Model file for the job. Use its own axes, mm. A direction names the side the tool comes from. Coordinates: 2 decimals unless noted, no trailing zeros. Loops run counter-clockwise (first coordinate to the right, second up) from the corner with the lowest first, then second, coordinate; pieces in that order, holes last. Notation, with made-up numbers: (79, 52) -> (131, 52) arc R18 cw to (131, 63) -> close; hole circle Ø5 at (33, 55). An arc over 180 degrees is marked (long way). Use one line per item in the form item = value.
```python
from build123d import *

# Parameters (mm, degrees)
EXTRUDE_1_DEPTH = 10
SHELL_2_T       = 3
FILLET_3_R      = 10
FILLET_4_R      = 3
SKETCH_2_R      = 2.675
EXTRUDE_2_DEPTH = 8
FILLET_7_R      = 5
CHAMFER_1_SIZE  = 0.2
CHAMFER_2_SIZE  = 0.2
FILLET_9_SIZE   = 5.5
FILLET_9_SIZE_2 = 5


# Some blends are built 0.0001 mm under size
with BuildPart() as part:
    # 草图1 → 凸台-拉伸1 (new body)
    with BuildSketch(Plane(origin=(0, 0, 0), x_dir=(1, 0, 0), z_dir=(0, 1, 0))):
        with BuildLine():
            Line((-37.5, 15), (37.5, 15))
            ThreePointArc((37.5, 15), (44.571067812, 12.071067812), (47.5, 5))
            Line((47.5, 5), (47.5, -5))
            ThreePointArc((47.5, -5), (44.571067812, -12.071067812), (37.5, -15))
            Line((37.5, -15), (-37.5, -15))
            ThreePointArc((-37.5, -15), (-44.571067812, -12.071067812), (-47.5, -5))
            Line((-47.5, -5), (-47.5, 5))
            ThreePointArc((-47.5, 5), (-44.571067812, 12.071067812), (-37.5, 15))
        make_face()
    extrude(amount=EXTRUDE_1_DEPTH)

    # 抽壳2
    shell_2_openings = [part.faces().sort_by_distance(p)[0] for p in [
        (0, 0, 0),
    ]]
    offset(amount=SHELL_2_T, openings=shell_2_openings, kind=Kind.INTERSECTION)

    # 圆角3
    # the kernel refuses this fillet: 10 mm, written as the material it takes off along each edge
    with BuildSketch(Plane(origin=(37.5, 13, 5), x_dir=(1, 0, 0), z_dir=(0, 0, -1))) as fillet_3_piece_1:
        with BuildLine():
            CenterArc((13 - FILLET_3_R, FILLET_3_R), FILLET_3_R, 270, 90)
            Line((13 - FILLET_3_R, 0), (13, 0))
            Line((13, 0), (13, FILLET_3_R))
        make_face()
    revolve(axis=Axis((37.5, 13, 5), (0, -1, 0)), revolution_arc=90, mode=Mode.SUBTRACT)
    with BuildSketch(Plane(origin=(50.5, 13, 5), x_dir=(0, -1, 0), z_dir=(0, 0, -1)), Plane(origin=(-50.5, 13, -5), x_dir=(0, -1, 0), z_dir=(0, 0, 1))) as fillet_3_piece_2:
        with BuildLine():
            CenterArc((FILLET_3_R, FILLET_3_R), FILLET_3_R, 180, 90)
            Line((0, FILLET_3_R), (0, 0))
            Line((0, 0), (FILLET_3_R, 0))
        make_face()
    extrude(amount=10, mode=Mode.SUBTRACT)
    with BuildSketch(Plane(origin=(37.5, 13, -5), x_dir=(0, 0, -1), z_dir=(-1, 0, 0))) as fillet_3_piece_3:
        with BuildLine():
            CenterArc((13 - FILLET_3_R, FILLET_3_R), FILLET_3_R, 270, 90)
            Line((13 - FILLET_3_R, 0), (13, 0))
            Line((13, 0), (13, FILLET_3_R))
        make_face()
    revolve(axis=Axis((37.5, 13, -5), (0, -1, 0)), revolution_arc=90, mode=Mode.SUBTRACT)
    with BuildSketch(Plane(origin=(37.5, 13, -18), x_dir=(0, -1, 0), z_dir=(-1, 0, 0)), Plane(origin=(-37.5, 13, 18), x_dir=(0, -1, 0), z_dir=(1, 0, 0))) as fillet_3_piece_4:
        with BuildLine():
            CenterArc((FILLET_3_R, FILLET_3_R), FILLET_3_R, 180, 90)
            Line((0, FILLET_3_R), (0, 0))
            Line((0, 0), (FILLET_3_R, 0))
        make_face()
    extrude(amount=75, mode=Mode.SUBTRACT)
    with BuildSketch(Plane(origin=(-37.5, 13, -5), x_dir=(-1, 0, 0), z_dir=(0, 0, 1))) as fillet_3_piece_5:
        with BuildLine():
            CenterArc((13 - FILLET_3_R, FILLET_3_R), FILLET_3_R, 270, 90)
            Line((13 - FILLET_3_R, 0), (13, 0))
            Line((13, 0), (13, FILLET_3_R))
        make_face()
    revolve(axis=Axis((-37.5, 13, -5), (0, -1, 0)), revolution_arc=90, mode=Mode.SUBTRACT)
    with BuildSketch(Plane(origin=(-37.5, 13, 5), x_dir=(0, 0, 1), z_dir=(1, 0, 0))) as fillet_3_piece_6:
        with BuildLine():
            CenterArc((13 - FILLET_3_R, FILLET_3_R), FILLET_3_R, 270, 90)
            Line((13 - FILLET_3_R, 0), (13, 0))
            Line((13, 0), (13, FILLET_3_R))
        make_face()
    revolve(axis=Axis((-37.5, 13, 5), (0, -1, 0)), revolution_arc=90, mode=Mode.SUBTRACT)

    # 圆角4
    fillet_4_edges = [part.edges().sort_by_distance(p)[0] for p in [
        (50.5, 0, 0),
        (46.692388155, 0, 14.192388155),
        (0, 0, 18),
        (-46.692388155, 0, 14.192388155),
        (-50.5, 0, 0),
        (-46.692388155, 0, -14.192388155),
        (0, 0, -18),
        (46.692388155, 0, -14.192388155),
    ]]
    fillet(fillet_4_edges, radius=FILLET_4_R - 0.0001)  # a hair under: the kernel refuses the full size

    # 草图2 → 凸台-拉伸2 (add)
    # profile 1 of 2: a face of its own
    with BuildSketch(Plane(origin=(0, 10, 0), x_dir=(-1, 0, 0), z_dir=(0, -1, 0))):
        with Locations(Location((36.8, 0, 0), (0, 0, 270))):
            Circle(SKETCH_2_R)
        Polygon((34.725, -0.575), (34.725, 0.575), (36.225, 0.575), (36.225, 2.075), (37.375, 2.075), (37.375, 0.575), (38.875, 0.575), (38.875, -0.575), (37.375, -0.575), (37.375, -2.075), (36.225, -2.075), (36.225, -0.575), align=None, mode=Mode.SUBTRACT)
    # profile 2 of 2: a face of its own
    with BuildSketch(Plane(origin=(0, 10, 0), x_dir=(-1, 0, 0), z_dir=(0, -1, 0))):
        with Locations(Location((-36.8, 0, 0), (0, 0, 90))):
            Circle(SKETCH_2_R)
        Polygon((-37.375, 0.575), (-37.375, 2.075), (-36.225, 2.075), (-36.225, 0.575), (-34.725, 0.575), (-34.725, -0.575), (-36.225, -0.575), (-36.225, -2.075), (-37.375, -2.075), (-37.375, -0.575), (-38.875, -0.575), (-38.875, 0.575), align=None, mode=Mode.SUBTRACT)
    extrude(amount=EXTRUDE_2_DEPTH)

    # 圆角7
    fillet_7_edges = [part.edges().sort_by_distance(p)[0] for p in [
        (-44.571067812, 10, 12.071067812),
        (0, 10, 15),
        (44.571067812, 10, 12.071067812),
        (47.5, 10, 0),
        (44.571067812, 10, -12.071067812),
        (0, 10, -15),
        (-44.571067812, 10, -12.071067812),
        (-47.5, 10, 0),
    ]]
    fillet(fillet_7_edges, radius=FILLET_7_R)

    # 倒角1
    chamfer_1_edges = [part.edges().sort_by_distance(p)[0] for p in [
        (35.475, 2, -0.575),
        (37.375, 2, 1.325),
        (38.875, 2, 0),
        (38.125, 2, -0.575),
        (37.375, 2, -1.325),
        (36.8, 2, -2.075),
        (34.725, 2, 0),
        (35.475, 2, 0.575),
        (36.225, 2, 1.325),
        (36.8, 2, 2.075),
        (38.125, 2, 0.575),
        (36.225, 2, -1.325),
    ]]
    chamfer(chamfer_1_edges, length=CHAMFER_1_SIZE)

    # 倒角2
    chamfer_2_edges = [part.edges().sort_by_distance(p)[0] for p in [
        (-36.8, 2, -2.075),
        (-37.375, 2, -1.325),
        (-38.125, 2, -0.575),
        (-38.875, 2, 0),
        (-37.375, 2, 1.325),
        (-35.475, 2, -0.575),
        (-38.125, 2, 0.575),
        (-36.8, 2, 2.075),
        (-36.225, 2, 1.325),
        (-35.475, 2, 0.575),
        (-34.725, 2, 0),
        (-36.225, 2, -1.325),
    ]]
    chamfer(chamfer_2_edges, length=CHAMFER_2_SIZE)

    # 圆角9
    # a fillet whose section is not a circle: 5.5, 5 mm, written as the material it adds along each edge
    with BuildSketch(Plane(origin=(36.8, 10, 0), x_dir=(0, 0, -1), z_dir=(-1, 0, 0))) as fillet_9_piece_1:
        with BuildLine():
            Bezier((2.675 + FILLET_9_SIZE, 0), (2.675, 0), (2.675, FILLET_9_SIZE_2), weights=[1, 0.333333333, 1])
            Line((2.675, FILLET_9_SIZE_2), (2.675, 0))
            Line((2.675, 0), (2.675 + FILLET_9_SIZE, 0))
        make_face()
    revolve(axis=Axis((36.8, 10, 0), (0, -1, 0)))

    # 圆角10
    # a fillet whose section is not a circle: 5.5, 5 mm, written as the material it adds along each edge (its section moved 0.00015 mm through the faces so that the kernel can cut it)
    with BuildSketch(Plane(origin=(-36.8, 10, 0), x_dir=(0, 0, 1), z_dir=(1, 0, 0))) as fillet_10_piece_1:
        with BuildLine():
            Bezier((7.675, -0.00015), (2.67485, -0.00015), (2.67485, 5.5), weights=[1, 0.333333333, 1])
            Line((2.67485, 5.5), (2.56485, 5.5))
            ThreePointArc((2.56485, 5.5), (2.565, 2.75), (2.565, 0))
            Line((2.565, 0), (2.675, -0.11))
            ThreePointArc((2.675, -0.11), (5.175, -0.11), (7.675, -0.11015))
            Line((7.675, -0.11015), (7.675, -0.00015))
        make_face()
    revolve(axis=Axis((-36.8, 10, 0), (0, -1, 0)))


solid = part.part
```
Q1. Which spindle directions (+Z, -Z, +X, -X, +Y, -Y) get a long thin tool onto all of the face, cutting with end or side? Do faces 3 (the face through (0.52, 0.86, -17.1)), 4 (the face through (-39.45, 3.28, -0.35)). Say none if no direction does.
Result:
face_3 = -Z, +X, -X, -Y
face_4 = -Y
Q2. Band-saw the part on C-C, the plane y = 1. Write the cut outline in (x, z), and give its area (3 significant figures).
Result:
outline = (-49.74, -5) arc R12.24 ccw to (-37.5, -17.24) -> (37.5, -17.24) arc R12.24 ccw to (49.74, -5) -> (49.74, 5) arc R12.24 ccw to (37.5, 17.24) -> (-37.5, 17.24) arc R12.24 ccw to (-49.74, 5) -> close; hole (-47.5, -5) arc R10 ccw to (-37.5, -15) -> (37.5, -15) arc R10 ccw to (47.5, -5) -> (47.5, 5) arc R10 ccw to (37.5, 15) -> (-37.5, 15) arc R10 ccw to (-47.5, 5) -> close
area = 536 mm2
Q3. Wall check: line 1 along Z through (x, y) = (-33, 9.25); line 2 along Z through (x, y) = (38, 4) (1 decimal); line 3 along Y through (x, z) = (27, 1.5). Give the ranges that are in metal, low to high.
Result:
line_1 = -15.81 to -12.63, -4.63 to 4.63, 12.63 to 15.81
line_2 = -17.9 to -15, -2.4 to -0.6, 0.6 to 2.4, 15 to 17.9
line_3 = 10 to 13
Q4. Band-saw the part on B-B, the plane y = 9. State how many separate pieces and enclosed holes the cut face has, and give its area (3 significant figures).
Result:
separate_pieces = 3
enclosed_holes = 3
area = 880 mm2
Q5. Mould opens along X. For faces 1 (the face through (1, 13, 0)), 2 (the face through (35.6, 2, -1.2)) say: released by +X, released by -X, zero draft, split by the parting line, or undercut.
Result:
face_1 = zero draft
face_2 = undercut
Q6. Pin check, flat tips, straight feed: pin 1 Ø1.2 at (x, y) = (38.5, 7) entering from -Z; pin 2 Ø0.9 at (y, z) = (7, 0) entering from -X; pin 3 Ø1.6 at (x, z) = (36.5, 0.5) entering from -Y. Stop position of each tip, or through.
Result:
pin_1 = -17.37
pin_2 = -49.85
pin_3 = 2
